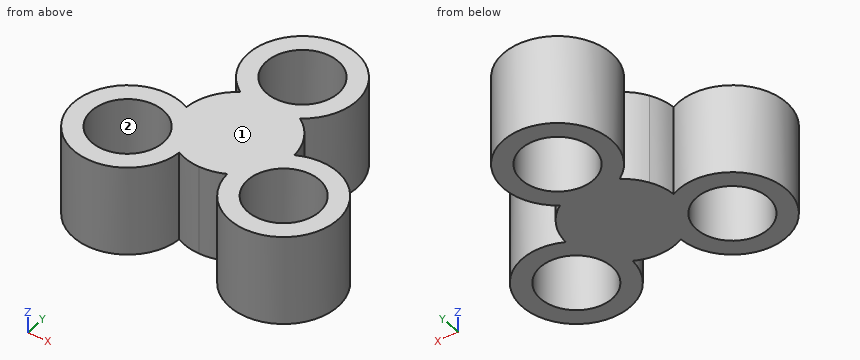
from build123d import *

# Parameters (mm, degrees)
F0_R     = 9.95
F1_DEPTH = 25


with BuildPart() as f1:
    # F0 (on Top) → F1 (new body)
    with BuildSketch(Plane.XY):
        with BuildLine():
            ThreePointArc((8.291562, 12.5), (0, 40), (-8.291562, 12.5))
            ThreePointArc((-8.291562, 12.5), (-10.930703, 10.272279), (-12.990381, 7.5))
            ThreePointArc((-12.990381, 7.5), (-14.361407, 4.330127), (-14.971099, 0.930703))
            ThreePointArc((-14.971099, 0.930703), (-34.641016, -20), (-6.679537, -13.430703))
            ThreePointArc((-6.679537, -13.430703), (-3.430703, -14.602406), (0, -15))
            ThreePointArc((0, -15), (3.430703, -14.602406), (6.679537, -13.430703))
            ThreePointArc((6.679537, -13.430703), (34.641016, -20), (14.971099, 0.930703))
            ThreePointArc((14.971099, 0.930703), (14.361407, 4.330127), (12.990381, 7.5))
            ThreePointArc((12.990381, 7.5), (10.930703, 10.272279), (8.291562, 12.5))
        make_face()
        with Locations((-21.650635, -12.5)):
            Circle(F0_R, mode=Mode.SUBTRACT)
        with Locations((21.650635, -12.5)):
            Circle(F0_R, mode=Mode.SUBTRACT)
        with Locations((0, 25)):
            Circle(F0_R, mode=Mode.SUBTRACT)
    extrude(amount=F1_DEPTH)


solid = f1.part
Build history of the part. All positions in model axes, mm. Face numbers are marked on the shaded views. Give positions to 0.01 mm unless a question says otherwise; leave off trailing zeros. Write each loop counter-clockwise with the first axis right and the second up, starting at its lowest first coordinate (ties: lowest second). Pieces come first, ordered by that corner, then holes. Notation, with made-up numbers: (29, -18.75) - (45, -18.75) arc R19 ccw to (45, -6.75) - close; hole circle Ø2 at (-8.75, 62.25). An arc over 180 degrees is marked (long way). Use one line per item in the form item = value. Start each with the question number.
1. Drop flat-ended pins along their axis: pin 1 Ø3 at (x, z) = (-27.5, 10) entering from -Y; pin 2 Ø3 at (y, z) = (11.5, 6) entering from +X; pin 3 Ø6 at (y, z) = (26, 7) entering from -X; pin 4 Ø12 at (x, y) = (0, 25) entering from -Z. Give the stop position or say it passes through.
2. Two-plate mould, pull along Y, no slides. Class the marked faces 1 and 2: released by +Y, released by -Y, zero draft, split by the parting line, or undercut.
3. Band-saw the part on C-C on y = 34. Write the cut outline in (x, z), plus the area to 3 significant figures.
4. Band-saw the part on A-A on y = -12.5. Write the cut outline in (x, z), plus the area to 3 significant figures.
5. Band-saw the part on D-D on x = 19. Write the cut outline in (y, z), plus the area to 3 significant figures.
6. Probe line 1 (Y direction, x = -0.5, z = 17); line 2 (X direction, y = -11.5, z = 16.25); line 3 (X direction, y = 24.5, z = 10.5). List the from-to ranges inside material, lowest first. Write a range as [from, to].
7. Band-saw the part on B-B on z = 9. Write the cut outline in (x, y).
Conclusion:
q1.pin_1 = -26.86
q1.pin_2 = 11.18
q1.pin_3 = -15
q1.pin_4 = through
q2.face_1 = zero draft
q2.face_2 = undercut
q3.outline = (-12, 0) - (-4.24, 0) - (-4.24, 25) - (-12, 25) - close; (4.24, 0) - (12, 0) - (12, 25) - (4.24, 25) - close
q3.area = 388 mm²
q4.outline = (-36.65, 0) - (-31.6, 0) - (-31.6, 25) - (-36.65, 25) - close; (-11.7, 0) - (11.7, 0) - (11.7, 25) - (-11.7, 25) - close; (31.6, 0) - (36.65, 0) - (36.65, 25) - (31.6, 25) - close
q4.area = 838 mm²
q5.outline = (-27.26, 0) - (-22.09, 0) - (-22.09, 25) - (-27.26, 25) - close; (-2.91, 0) - (2.26, 0) - (2.26, 25) - (-2.91, 25) - close
q5.area = 259 mm²
q6.line_1 = [-14.99, 15.06], [34.94, 39.99]
q6.line_2 = [-36.62, -31.55], [-11.75, 11.75], [31.55, 36.62]
q6.line_3 = [-14.99, -9.94], [9.94, 14.99]
q7.outline = (-14.97, 0.93) arc R15 ccw (long way) to (-6.68, -13.43) arc R15 ccw to (0, -15) arc R15 ccw to (6.68, -13.43) arc R15 ccw (long way) to (14.97, 0.93) arc R15 ccw to (12.99, 7.5) arc R15 ccw to (8.29, 12.5) arc R15 ccw (long way) to (-8.29, 12.5) arc R15 ccw to (-12.99, 7.5) arc R15 ccw to start; hole circle Ø19.9 at (-21.65, -12.5); hole circle Ø19.9 at (0, 25); hole circle Ø19.9 at (21.65, -12.5)
